Could you check a few things on this model? Use its own coordinates, in mm. Round coordinates to 2 decimals unless told otherwise and drop trailing zeros. Write each loop counter-clockwise with the first axis right and the second up, starting at its lowest first coordinate (ties: lowest second). Pieces come first, ordered by that corner, then holes. Notation, with made-up numbers: (-18, -5) -> (32, -5) arc R8 cw to (32, 10) -> close; hole circle Ø1 at (-15, 39). An arc over 180 degrees is marked (long way). Answer in a Markdown table with one row per item.
from build123d import *

# Parameters (mm, degrees)
SKETCH1_R           = 1.2
BOSS_EXTRUDE1_DEPTH = 3.5
FILLET1_R           = 0.5


with BuildPart() as part:
    # Sketch1 → Boss-Extrude1 (new body)
    with BuildSketch(Plane(origin=(0, 0, 0), x_dir=(1, 0, 0), z_dir=(0, 1, 0))):
        with BuildLine():
            Line((0, 0), (0, -5.17))
            Line((0, -5.17), (18, -5.17))
            Line((18, -5.17), (18, 0))
            ThreePointArc((18, 0), (9, 2.577794898), (0, 0))
        make_face()
        with Locations(Location((4, -0.17, 0), (0, 0, 270))):
            Circle(SKETCH1_R, mode=Mode.SUBTRACT)
        with Locations(Location((14, -0.17, 0), (0, 0, 270))):
            Circle(SKETCH1_R, mode=Mode.SUBTRACT)
    extrude(amount=BOSS_EXTRUDE1_DEPTH)

    # Fillet1
    fillet1_edges = [part.edges().sort_by_distance(p)[0] for p in [
        (0, 3.5, 2.585),
        (9, 3.5, 5.17),
        (18, 3.5, 2.585),
        (9, 0, 5.17),
        (0, 0, 2.585),
        (9, 0, -2.577794898),
        (18, 0, 2.585),
        (18, 1.75, 5.17),
        (0, 1.75, 5.17),
        (0, 1.75, 0),
        (18, 1.75, 0),
        (9, 3.5, -2.577794898),
    ]]
    fillet(fillet1_edges, radius=FILLET1_R)


solid = part.part
1) For pin 1 (4 mm diameter, centred on x = 4, z = 0.17, fed in from +Y); pin 2 (1 mm diameter, centred on x = 10, y = 0.5, fed in from -Z), each with a flat end and sliding along its axis, tell me the tip position at first contact or that it passes through.
Findings:
| item | result |
|---|---|
| pin 1 | stops at y = 3.5 |
| pin 2 | stops at z = -2.57 |
2) Imagine slicing it at B-B, the plane z = 0.5. Please give me the cut outline in (x, y), plus the area to 3 significant figures.
Findings:
| item | result |
|---|---|
| outline | (0, 0.5) arc R0.5 ccw to (0.5, 0) -> (2.85, 0) -> (2.85, 3.5) -> (0.5, 3.5) arc R0.5 ccw to (0, 3) -> close; (5.15, 0) -> (12.85, 0) -> (12.85, 3.5) -> (5.15, 3.5) -> close; (15.15, 0) -> (17.5, 0) arc R0.5 ccw to (18, 0.5) -> (18, 3) arc R0.5 ccw to (17.5, 3.5) -> (15.15, 3.5) -> close |
| area | 46.6 mm^2 |
3) Imagine slicing it at C-C, the plane y = 0.3. Please give me the cut outline in (x, z).
Findings:
| item | result |
|---|---|
| outline | (0.04, 0.28) arc R0.46 ccw to (0.26, -0.11) arc R16.96 ccw to (17.74, -0.11) arc R0.46 ccw to (17.96, 0.28) -> (17.96, 4.67) arc R0.46 ccw to (17.5, 5.13) -> (0.5, 5.13) arc R0.46 ccw to (0.04, 4.67) -> close; hole circle Ø2.4 at (4, 0.17); hole circle Ø2.4 at (14, 0.17) |
4) Imagine slicing it at A-A, the plane y = 1.4. Please give me the cut outline in (x, z).
Findings:
| item | result |
|---|---|
| outline | (0, 0.28) arc R0.5 ccw to (0.24, -0.15) arc R17 ccw to (17.76, -0.15) arc R0.5 ccw to (18, 0.28) -> (18, 4.67) arc R0.5 ccw to (17.5, 5.17) -> (0.5, 5.17) arc R0.5 ccw to (0, 4.67) -> close; hole circle Ø2.4 at (4, 0.17); hole circle Ø2.4 at (14, 0.17) |
5) Please list where these lines run through material, in increasing order: line 1 (X direction, y = 0.6, z = 0.25); line 2 (X direction, y = 1.35, z = -0.5); line 3 (Z direction, x = 4.5, y = 2.6).
Findings:
| item | result |
|---|---|
| line 1 | x = 0 to 2.8, 5.2 to 12.8, 15.2 to 18 |
| line 2 | x = 0.86 to 3, 5 to 13, 15 to 17.14 |
| line 3 | z = -1.97 to -0.92, 1.26 to 5.17 |
6) Thinking about a two-plate mould opening in X: for faces 1 (the face through (9.129, 1.732, -2.577)), 2 (the face through (9, 0, 2)), 3 (the face through (12.83, 1.73, -0.09)), 4 (the face through (18, 2, 3)), which applies, +X half, -X half, draft (parallel to the pull), parting line (faces both ways), or undercut?
Findings:
| item | result |
|---|---|
| face 1 | parting line |
| face 2 | draft |
| face 3 | undercut |
| face 4 | +X half |
